Work out the finished part from the listing and answer in its coordinate system (mm). A direction names the side the tool comes from. Coordinates: 2 decimals unless noted, no trailing zeros. Order: outer loops, then holes, each group sorted by start corner. A loop starts at its lowest first (then second) coordinate and runs counter-clockwise, first axis right, second up. Notation, with made-up numbers: M 64,13 L 87,13 A31 cw 87,44 Z; hole C 38,80.25 d3. An arc over 180 degrees is marked long. Write item = value, one per line. Start each with the question number.
Q1. A tool of negligible diameter and unlimited length cuts with its end or side. For faces 1 (the flat face through (8, 6, -7.8)), 2 (the cylindrical face through (13.924, 3.989, -2.61)), 3 (the flat face through (8, 1, -1.2)), from which of +Z, -Z, +X, -X, +Y, -Y can it reach the whole face along a straight path? Write none if from no direction.
Q2. Find section D-D on y = 6.75. Give the vertices of the cut face in (x, z).
Q3. Find section C-C on x = 7.9. Give the vertices of the cut face in (y, z), and give its area (3 significant figures).
Q4. Each of these flat-tipped pins is pushed along its axis until it touches: P1, Ø1.6, axis at x = 11.5, y = 4.5, coming from the -Z side; P2, Ø3, axis at x = 5.5, z = -4, coming from the +Y side; P3, Ø1.9, axis at x = 7.9, z = -3.9, coming from the +Y side. Where does it stop, or does it pass through?
Q5. Find section A-A on y = 4. Give the vertices of the cut face in (x, z).
Q6. Straight lines are drawn through the part: line 1 along Z through (x, y) = (7, 1.5); line 2 along Z through (x, y) = (11.9, 2.65); line 3 along Z through (x, y) = (2.25, 1.5). For each, find the intervals that lie inside material, in ascending order.
Q7. Determine the mould class of faces 4 (the flat face through (4, 3.6, -4)), 5 (the cylindrical face through (3.139, 2.536, -9.889)) for opening direction Z: released by +Z, released by -Z, zero draft, split by the parting line, or undercut.
```python
from build123d import *

# Parameters (mm, degrees)
SKETCH1_W            = 15.8
SKETCH1_H            = 3.2
BOSS_EXTRUDE1_DEPTH  = 7.8
SKETCH2_R            = 2.4
BOSS_EXTRUDE2_DEPTH  = 1.6
LPATTERN1_COUNT      = 2
LPATTERN1_PITCH      = 8
LPATTERN1_COUNT_DIR2 = 4
LPATTERN1_PITCH_DIR2 = 8
SHELL1_T             = -1.2
SKETCH3_R            = 1.5
SKETCH3_R_2          = 0.6
BOSS_EXTRUDE3_DEPTH  = 1.8
SKETCH4_W            = 15.8
SKETCH4_H            = 7.9
BOSS_EXTRUDE4_DEPTH  = 1.3
SKETCH5_R            = 2.35
SKETCH5_R_2          = 1.65
BOSS_EXTRUDE5_DEPTH  = 1.6
LPATTERN2_COUNT      = 2
LPATTERN2_PITCH      = 8


with BuildPart() as part:
    # Sketch1 → Boss-Extrude1 (new body)
    with BuildSketch(Plane.XY):
        with Locations((7.9, 1.6)):
            Rectangle(SKETCH1_W, SKETCH1_H)
    extrude(amount=-BOSS_EXTRUDE1_DEPTH)

    # Sketch2 → Boss-Extrude2 (add)
    with BuildSketch(Plane(origin=(0, 3.2, 0), x_dir=(1, 0, 0), z_dir=(0, 1, 0))):
        with Locations(Location((3.9, 3.9, 0), (0, 0, 270))):
            Circle(SKETCH2_R)
    boss_extrude2 = extrude(amount=BOSS_EXTRUDE2_DEPTH)

    # LPattern1: Boss-Extrude2 2 × 4, 6 skipped
    with Locations(*[(j * LPATTERN1_PITCH_DIR2, 0, i * LPATTERN1_PITCH) for i in range(LPATTERN1_COUNT) for j in range(LPATTERN1_COUNT_DIR2) if (i, j) not in ((0, 0), (0, 2), (0, 3), (1, 0), (1, 1), (1, 2), (1, 3))]):
        add(boss_extrude2)

    # Shell1
    shell1_openings = [part.faces().sort_by_distance(p)[0] for p in [
        (7.9, 0, -3.9),
    ]]
    offset(amount=SHELL1_T, openings=shell1_openings, kind=Kind.INTERSECTION)

    # Sketch3 → Boss-Extrude3 (add)
    with BuildSketch(Plane.XZ.offset(-2)):
        with Locations(Location((7.9, -3.9, 0), (0, 0, 90))):
            Circle(SKETCH3_R)
        with Locations(Location((7.9, -3.9, 0), (0, 0, 270))):
            Circle(SKETCH3_R_2, mode=Mode.SUBTRACT)
    extrude(amount=BOSS_EXTRUDE3_DEPTH)

    # Sketch4 → Boss-Extrude4 (add)
    with BuildSketch(Plane(origin=(0, 0, -7.8), x_dir=(-1, 0, 0), z_dir=(0, 0, -1))):
        with Locations((-7.9, 3.95)):
            Rectangle(SKETCH4_W, SKETCH4_H)
    extrude(amount=BOSS_EXTRUDE4_DEPTH)

    # Sketch5 → Boss-Extrude5 (add)
    with BuildSketch(Plane(origin=(0, 0, -9.1), x_dir=(-1, 0, 0), z_dir=(0, 0, -1))):
        with Locations(Location((-11.9, 4, 0), (0, 0, 180))):
            Circle(SKETCH5_R)
        with Locations((-11.9, 4)):
            Circle(SKETCH5_R_2, mode=Mode.SUBTRACT)
    boss_extrude5 = extrude(amount=BOSS_EXTRUDE5_DEPTH)

    # LPattern2: Boss-Extrude5 ×2
    with Locations(*[(-i * LPATTERN2_PITCH, 0, 0) for i in range(1, LPATTERN2_COUNT)]):
        add(boss_extrude5)


solid = part.part
```
Findings below:
q1.face_1 = +X, -X, +Y
q1.face_2 = +Y
q1.face_3 = -Y
q2.outline = M 0,-9.1 L 15.8,-9.1 L 15.8,-7.8 L 0,-7.8 Z
q3.outline = M 0,-9.1 L 7.9,-9.1 L 7.9,-7.8 L 3.2,-7.8 L 3.2,0 L 0,0 L 0,-1.2 L 2,-1.2 L 2,-2.4 L 0.2,-2.4 L 0.2,-3.3 L 2,-3.3 L 2,-4.5 L 0.2,-4.5 L 0.2,-5.4 L 2,-5.4 L 2,-6.6 L 0,-6.6 Z
q3.area = 27.7 mm^2
q4.P1 = -9.1
q4.P2 = 4.8
q4.P3 = 3.2
q5.outline = M 0,-9.1 L 1.55,-9.1 L 1.55,-10.7 L 2.25,-10.7 L 2.25,-9.1 L 5.55,-9.1 L 5.55,-10.7 L 6.25,-10.7 L 6.25,-9.1 L 9.55,-9.1 L 9.55,-10.7 L 10.25,-10.7 L 10.25,-9.1 L 13.55,-9.1 L 13.55,-10.7 L 14.25,-10.7 L 14.25,-9.1 L 15.8,-9.1 L 15.8,-7.8 L 0,-7.8 Z; C 3.9,-3.9 d4.8; C 11.9,-3.9 d4.8
q6.line_1 = -9.1 to -6.6, -5.1 to -2.7, -1.2 to 0
q6.line_2 = -9.1 to -5.1, -2.7 to 0
q6.line_3 = -9.1 to -6.6, -1.2 to 0
q7.face_4 = undercut
q7.face_5 = zero draft
